CAD build for the part. Positions are in the model's coordinates, mm. A direction names the side the tool comes from. Give positions to 0.01 mm unless a question says otherwise; leave off trailing zeros. Write each loop counter-clockwise with the first axis right and the second up, starting at its lowest first coordinate (ties: lowest second). Pieces come first, ordered by that corner, then holes. Notation, with made-up numbers: (85.5, 35.5) -> (142.5, 35.5) arc R29 ccw to (142.5, 64.5) -> close; hole circle Ø5 at (55, 51). An arc over 180 degrees is marked (long way). Answer as a JSON object with one key per item and string values.
Autodesk Inventor part; units mm, degrees
ref_plane "Start Plane" through (0, 0, 0) normal (1, 0, 0) x (0, 1, 0)
ref_plane "XZ Plane" through (0, 0, 0) normal (0, 1, 0) x (-1, 0, 0)
ref_plane "XY Plane" through (0, 0, 0) normal (0, 0, 1) x (1, 0, 0)
sketch "Main Sketch" plane through (0, 0, 0) normal (0, 0, 1) x (1, 0, 0)
  line L0 (0, 0) -> (7.95, 0)
  line L1 (0, 0) -> (0, 0.625)
  line L2 (3.45, 0.5) -> (3.45, 0.625)
  line L3 (0, 0.625) -> (0.25, 0.625)
  line L4 (3.95, 0.625) -> (3.95, 0.5)
  line L5 (3.45, 0.625) -> (3.95, 0.625)
  line L6 (7.45, 0.25) -> (7.45, 0.75)
  line L7 (6.95, 0.25) -> (7.45, 0.25)
  line L8 (7.95, 0.75) -> (7.95, 0)
  line L9 (7.45, 0.75) -> (7.95, 0.75)
  line L10 (0.25, 0.625) -> (0.25, 0.5)
  line L11 (0.25, 0.5) -> (3.45, 0.5)
  line L12 (3.7, 0.375) -> (6.2, 0.375)
  line L13 (6.2, 0.375) -> (6.2, 0.5)
  line L14 (6.7, 0.5) -> (6.7, 0.25)
  line L15 (6.2, 0.5) -> (6.7, 0.5)
  line L16 (3.95, 0.5) -> (6.45, 0.5)
  line L17 (6.45, 0.5) -> (6.45, 0.625)
  line L18 (6.95, 0.625) -> (6.95, 0.25)
  line L19 (6.45, 0.625) -> (6.95, 0.625)
  dimension "d3" = 1.25
  dimension "d6" = 1.25
  dimension "d7" = 0.5
  dimension "d10" = 1.5
  dimension "d15" = 1
  dimension "d22" = 0.75
  dimension "d23" = 1
  dimension "d24" = 1
  dimension "d25" = 1.25
revolve "Revolution1" add sketch "Main Sketch" angle 360 about axis through (0, 0, 0) along (1, 0, 0)
chamfer "Chamfer3" [suppressed]
chamfer "Chamfer1" distance 0.25 angle 45 1 edges at (7.95, -0.75, 0) measured on face at (7.6167, 0.7476, -0.0603)
equation "\"Length\" = 7.95"
properties part number "Shaft" material "Steel"
1) Slice it at C-C (x = 2.5). List the corners of the cut face in (y, z), then the cut area to 3 significant figures.
Model answer:
{"outline": "circle Ø1 at (0, 0)", "area": "0.785 mm2"}
2) Mould opens along X. For faces 3 (the cylindrical face through (5.218, -0.108, -0.488)), 4 (the flat face through (7.95, 0, 0)), 5 (the cylindrical face through (6.7, -0.14, -0.61)), 6 (the flat face through (0, 0, 0)) say: released by +X, released by -X, zero draft, split by the parting line, or undercut.
Model answer:
{"face 3": "undercut", "face 4": "released by +X", "face 5": "zero draft", "face 6": "released by -X"}
3) 3-axis set-ups, long thin cutter, end or side, ignore diameter. For faces 1 (the cylindrical face through (1.872, -0.108, -0.488)), 2 (the cylindrical face through (3.7, -0.14, -0.61)): which of +Z, -Z, +X, -X, +Y, -Y reach the whole face in a straight line?
Model answer:
{"face 1": "none", "face 2": "-X"}
4) Wall check: probe 1 along X at (y, z) = (-0.35, 0.05); probe 2 along X at (y, z) = (0.3, -0.5); probe 3 along Z at (x, y) = (3.25, 0.05). Give the ranges that are in metal, low to high.
Model answer:
{"probe 1": "x = 0 to 6.95, 7.45 to 7.95", "probe 2": "x = 0 to 0.25, 3.45 to 3.95, 6.45 to 6.95, 7.45 to 7.87", "probe 3": "z = -0.5 to 0.5"}
